Autodesk Fusion 360 part; units mm, degrees
sketch "スケッチ1" plane through (0, 0, 0) normal (0, 0, 1) x (1, 0, 0)
  circle A0 centre (0, 0) radius 50
extrude "押し出し1" add sketch "スケッチ1" along normal blind 10
sketch "スケッチ2" plane through (0, 0, 10) normal (0, 0, 1) x (1, 0, 0)
  circle A0 centre (0, 0) radius 50
  circle A1 centre (0, 40) radius 4.7499
extrude "押し出し2" cut sketch "スケッチ2" against normal blind 10 contours A1
sketch "スケッチ3" plane through (0, 0, 10) normal (0, 0, 1) x (1, 0, 0)
  circle A0 centre (0, 40) radius 4.7499
  circle A1 centre (0, 0) radius 50
sketch "スケッチ4" plane through (0, 0, 10) normal (0, 0, 1) x (1, 0, 0)
sketch "スケッチ5" plane through (0, 0, 10) normal (0, 0, 1) x (1, 0, 0)
sketch "スケッチ6" plane through (0, 0, 10) normal (0, 0, 1) x (1, 0, 0)
sketch "スケッチ7" plane through (0, 0, 10) normal (0, 0, 1) x (1, 0, 0)
sketch "スケッチ8" plane through (0, 0, 10) normal (0, 0, 1) x (1, 0, 0)
sketch "スケッチ9" plane through (0, 0, 10) normal (0, 0, 1) x (1, 0, 0)
sketch "スケッチ10" plane through (0, 0, 10) normal (0, 0, 1) x (1, 0, 0)
sketch "スケッチ11" plane through (0, 0, 10) normal (0, 0, 1) x (1, 0, 0)
sketch "スケッチ12" plane through (0, 0, 10) normal (0, 0, 1) x (1, 0, 0)
sketch "スケッチ13" plane through (0, 0, 10) normal (0, 0, 1) x (1, 0, 0)
sketch "スケッチ14" plane through (0, 0, 10) normal (0, 0, 1) x (1, 0, 0)
  line L0 (-25, 25) -> (-15, 25)
  line L1 (-15, 25) -> (-15, -30)
  line L2 (-15, -30) -> (-25, -30)
  line L3 (-25, -30) -> (-25, 25)
  line L4 (0, 25) -> (35, 25)
  line L5 (35, 25) -> (35, 15)
  line L6 (35, 15) -> (0, 15)
  line L7 (0, 15) -> (0, 25)
  line L8 (10, 15) -> (25, 15)
  line L9 (25, 15) -> (25, -30)
  line L10 (25, -30) -> (10, -30)
  line L11 (10, -30) -> (10, 15)
extrude "押し出し3" add sketch "スケッチ14" sketch "スケッチ3" along normal blind 10 contours L0 L1 L2 L3 of sketch 2
sketch "スケッチ15" plane through (0, 0, 20) normal (0, 0, 1) x (1, 0, 0)
  circle A0 centre (0, 40) radius 4.7499
  circle A1 centre (0, 0) radius 50
  line L0 (-25, 25) -> (-15, 25)
  line L1 (-15, 25) -> (-15, -25)
  line L2 (-15, -25) -> (-25, -25)
  line L3 (-25, -25) -> (-25, 25)
  line L4 (0, 25) -> (25, 25)
  line L5 (25, 25) -> (25, 15)
  line L6 (25, 15) -> (0, 15)
  line L7 (0, 15) -> (0, 25)
  line L8 (10, 15) -> (15, 15)
  line L9 (15, 15) -> (15, -25)
  line L10 (15, -25) -> (10, -25)
  line L11 (10, -25) -> (10, 15)
extrude "押し出し4" add sketch "スケッチ15" along normal blind 10 contours L0 L1 L2 L3
sketch "スケッチ16" plane through (0, 0, 20) normal (0, 0, 1) x (1, 0, 0)
  line L0 (-25, -25) -> (-25, 25)
  line L1 (-25, 25) -> (-15, 25)
  line L2 (-15, 25) -> (-15, -25)
  line L3 (-15, -25) -> (-25, -25)
  circle A0 centre (0, 40) radius 4.7499
  circle A1 centre (0, 0) radius 50
  line L4 (0, 25) -> (35, 25)
  line L5 (35, 25) -> (35, 15)
  line L6 (35, 15) -> (0, 15)
  line L7 (0, 15) -> (0, 25)
  line L8 (10, 15) -> (25, 15)
  line L9 (25, 15) -> (25, -25)
  line L10 (25, -25) -> (10, -25)
  line L11 (10, -25) -> (10, 15)
extrude "押し出し5" add sketch "スケッチ16" along normal blind 10 contours L4 L5 L6 L7 L8 | L6 L8 L9 L10 L11
The listing builds one solid part. Answer for the finished solid, in the listing's coordinates (mm). A direction names the side the tool comes from. Give positions to 0.01 mm unless a question says otherwise; leave off trailing zeros. Loops run counter-clockwise (first coordinate to the right, second up) from the corner with the lowest first, then second, coordinate; pieces in that order, holes last.
Item 1: A cutting plane is placed at C-C (x = 1.5). Give the vertices of the cut face in (y, z).
Derived:
outline: (-49.98, 0) - (35.49, 0) - (35.49, 20) - (25, 20) - (25, 30) - (15, 30) - (15, 20) - (-49.98, 20) - close; (44.51, 0) - (49.98, 0) - (49.98, 20) - (44.51, 20) - close
Item 2: A cutting plane is placed at B-B (z = 24.25). Give the vertices of the cut face in (x, y), then the cut area to 3 significant figures.
Derived:
outline: (-25, -25) - (-15, -25) - (-15, 25) - (-25, 25) - close; (0, 15) - (10, 15) - (10, -25) - (25, -25) - (25, 15) - (35, 15) - (35, 25) - (0, 25) - close
area: 1,450 mm2
Item 3: A cutting plane is placed at A-A (y = 40). Give the vertices of the cut face in (x, z), then the cut area to 3 significant figures.
Derived:
outline: (-30, 0) - (-4.75, 0) - (-4.75, 20) - (-30, 20) - close; (4.75, 0) - (30, 0) - (30, 20) - (4.75, 20) - close
area: 1,010 mm2
Item 4: A tool of negligible diameter and unlimited length cuts with its end or side. For faces 4 (the flat face through (-20, 25, 25)), 5 (the flat face through (35, 20, 25)), 6 (the flat face through (30, 15, 25)), from which of +Z, -Z, +X, -X, +Y, -Y can it reach the whole face along a straight path? Write none if from no direction.
Derived:
face 4: +Z, +X, -X, +Y
face 5: +Z, +X, +Y, -Y
face 6: +Z, +X, -Y
Item 5: Find the intervals of material crossed by line 1 along Y through (x, z) = (0, 10.5); line 2 along X through (y, z) = (-3.5, 21); line 3 along Z through (x, y) = (45.5, 15), in increasing order.
Derived:
line 1: y = -50 to 35.25, 44.75 to 50
line 2: x = -25 to -15, 10 to 25
line 3: z = 0 to 20
Item 6: A cutting plane is placed at D-D (y = 0). Give the vertices of the cut face in (x, z).
Derived:
outline: (-50, 0) - (50, 0) - (50, 20) - (25, 20) - (25, 30) - (10, 30) - (10, 20) - (-15, 20) - (-15, 30) - (-25, 30) - (-25, 20) - (-50, 20) - close
Item 7: Each of these flat-tipped pins is pushed along its axis until it touches: pin 1 Ø5 at (y, z) = (22, 26) entering from -X; pin 2 Ø3 at (y, z) = (21.5, 26.5) entering from +X; pin 3 Ø5 at (x, z) = (-17.5, 27) entering from -Y. Where does it stop, or does it pass through?
Derived:
pin 1: stops at x = -25
pin 2: stops at x = 35
pin 3: stops at y = -25
Item 8: Determine the mould class of faces 1 (the flat face through (0, 20, 25)), 2 (the flat face through (17, 25, 25)), 3 (the flat face through (-25, 0, 25)) for opening direction X: +X half, -X half, draft (parallel to the pull), parting line (faces both ways), or undercut.
Derived:
face 1: undercut
face 2: draft
face 3: -X half
